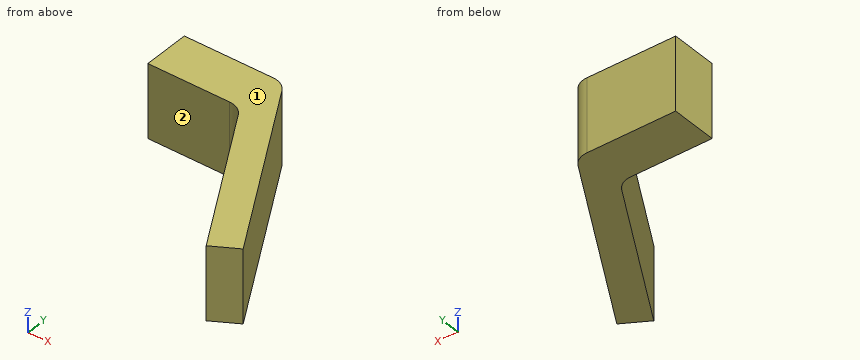
```python
from build123d import *

# Parameters (mm, degrees)
BOSS_EXTRUDE1_DEPTH = 15.875
FILLET1_R           = 4


with BuildPart() as part:
    # Sketch1 → Boss-Extrude1 (new body)
    with BuildSketch(Plane.XY):
        Polygon((-10, 0), (10, 0), (30, -34.641016151), (35.499261314, -31.466016151), (11.558845727, 10), (-10, 10), align=None)
    extrude(amount=BOSS_EXTRUDE1_DEPTH)

    # Fillet1
    fillet1_edges = [part.edges().sort_by_distance(p)[0] for p in [
        (11.558845727, 10, 7.9375),
        (10, 0, 7.9375),
    ]]
    fillet(fillet1_edges, radius=FILLET1_R)


solid = part.part
```
Could you check a few things on this model? Use its own coordinates, in mm. Face numbers are marked on the shaded views. A direction names the side the tool comes from. Round coordinates to 2 decimals unless told otherwise and drop trailing zeros. Loops run counter-clockwise (first coordinate to the right, second up) from the corner with the lowest first, then second, coordinate; pieces in that order, holes last. Notation, with made-up numbers: (-11, 72.5) - (34, 72.5) arc R20 cw to (34, 99.5) - close; hole circle Ø2 at (32, 30.5). An arc over 180 degrees is marked (long way). Use CSV: the item, a comma, the result in double quotes.
Item 1: If we section it at A-A on z = 9.25: List the corners of the cut face in (x, y) for me.
Here are the results:
outline,"(-10, 0) - (7.69, 0) arc R4 cw to (11.15, -2) - (30, -34.64) - (35.5, -31.47) - (12.71, 8) arc R4 ccw to (9.25, 10) - (-10, 10) - close"
Item 2: If we section it at C-C on y = 2: List the corners of the cut face in (x, z) for me (3 decimals).
Here are the results:
outline,"(-10, 0) - (16.178, 0) - (16.178, 15.875) - (-10, 15.875) - close"
Item 3: I need wall thicknesses on L1, parallel to Y at x = 6.5, z = 9.5; L2, parallel to X at y = -1.5, z = 12.5; L3, parallel to Y at x = 24.5, z = 3.25. Which ranges of each line are inside material? Lowest first, please. Write a range as [from, to].
Here are the results:
L1,"y = [0, 10]"
L2,"x = [10.81, 18.2]"
L3,"y = [-25.11, -12.41]"
Item 4: If we section it at B-B on x = -6.5: List the corners of the cut face in (y, z) for me (3 decimals), then the cut area to 3 significant figures.
Here are the results:
outline,"(0, 0) - (10, 0) - (10, 15.875) - (0, 15.875) - close"
area,"159 mm²"
Item 5: Will these pins go through, and if not, where does the flat tip stop? pin 1 (5 mm diameter, centred on x = 0.5, z = 11.5, fed in from -Y); pin 2 (5 mm diameter, centred on x = 14.5, z = 5.5, fed in from -Y); pin 3 (6 mm diameter, centred on y = -9.5, z = 6.5, fed in from -X).
Here are the results:
pin 1,"stops at y = 0"
pin 2,"stops at y = -12.12"
pin 3,"stops at x = 13.75"
Item 6: For the marked faces 1 and 2, which set-ups out of +Z, -Z, +X, -X, +Y, -Y let a thin tool reach every point of the face, with its end or its side?
Here are the results:
face 1,"+Z, +X, -X, +Y, -Y"
face 2,"+Z, -Z, -X, -Y"
